```python
from build123d import *

# Parameters (mm, degrees)
F1_DEPTH = 30
F2_R     = 5
F3_DEPTH = 28.448
F5_DEPTH = 25.4


with BuildPart() as f1:
    # F0 (on Front) → F1 (new body, symmetric)
    with BuildSketch(Plane.XZ):
        Polygon((-30, 0), (0, 0), (0, 60), (-10, 60), (-10, 10), (-30, 10), align=None)
    extrude(amount=F1_DEPTH, both=True)

    # F2 (on face) → F3 (cut)
    with BuildSketch(Plane.YZ):
        with Locations((0, 45)):
            Circle(F2_R)
    extrude(amount=-F3_DEPTH, mode=Mode.SUBTRACT)

    # F4 (on face) → F5 (cut)
    with BuildSketch(Plane.XY.offset(10)):
        with BuildLine():
            Line((-25, 5), (-30, 5))
            Line((-30, 5), (-30, -5))
            Line((-30, -5), (-25, -5))
            ThreePointArc((-25, -5), (-20, 0), (-25, 5))
        make_face()
    extrude(amount=-F5_DEPTH, mode=Mode.SUBTRACT)


solid = f1.part
```
Could you check a few things on this model? Use its own coordinates, in mm. A direction names the side the tool comes from. Round coordinates to 2 decimals unless told otherwise and drop trailing zeros. Write each loop counter-clockwise with the first axis right and the second up, starting at its lowest first coordinate (ties: lowest second). Pieces come first, ordered by that corner, then holes.
(1) Suppose I cut it at A-A on x = -26. Write out the boundary of the cut face in (y, z), and give its area (3 significant figures).
Findings below:
outline: (-30, 0) - (-5, 0) - (-5, 10) - (-30, 10) - close; (5, 0) - (30, 0) - (30, 10) - (5, 10) - close
area: 500 mm2
(2) For pin 1 (1.5 mm diameter, centred on y = 10, z = 53, fed in from -X); pin 2 (10 mm diameter, centred on x = -20.5, y = 1.5, fed in from +Z), each with a flat end and sliding along its axis, tell me the tip position at first contact or that it passes through.
Findings below:
pin 1: stops at x = -10
pin 2: stops at z = 10
(3) Thinking about a two-plate mould opening in Y: for faces 4 (the face through (-4.93, -0.651, 49.957)), 5 (the face through (-10, 0, 35)), 6 (the face through (-9, 30, 24)), which applies, +Y half, -Y half, draft (parallel to the pull), parting line (faces both ways), or undercut?
Findings below:
face 4: undercut
face 5: draft
face 6: +Y half
(4) If I drill on probe 1 along Z at (x, y) = (-5.5, 0); probe 2 along X at (y, z) = (23, 38); probe 3 along Z at (x, y) = (-24.25, 5.5), over which ranges is the centre line in solid material (lowest first)?
Findings below:
probe 1: z = 0 to 40, 50 to 60
probe 2: x = -10 to 0
probe 3: z = 0 to 10
(5) Suppose I cut it at D-D on x = -5. Write out the boundary of the cut face in (y, z).
Findings below:
outline: (-30, 0) - (30, 0) - (30, 60) - (-30, 60) - close; hole circle Ø10 at (0, 45)
(6) Suppose I cut it at C-C on z = 45. Write out the boundary of the cut face in (x, y).
Findings below:
outline: (-10, -30) - (0, -30) - (0, -5) - (-10, -5) - close; (-10, 5) - (0, 5) - (0, 30) - (-10, 30) - close
(7) Suppose I cut it at B-B on y = 4. Write out the boundary of the cut face in (x, z), and give its area (3 significant figures).
Findings below:
outline: (-22, 0) - (0, 0) - (0, 42) - (-10, 42) - (-10, 10) - (-22, 10) - close; (-10, 48) - (0, 48) - (0, 60) - (-10, 60) - close
area: 660 mm2
(8) Which directions (+Z, -Z, +X, -X, +Y, -Y) give clear straight access to the entire face, cutting with the end or side of a thin tool? Please do faces 1 (the face through (-19.86, -0.42, 10)), 2 (the face through (-9, -30, 24)), 3 (the face through (-28, -5, 5)).
Findings below:
face 1: +Z, -X, +Y, -Y
face 2: +Z, -Z, +X, -X, -Y
face 3: +Z, -Z, -X
